Autodesk Inventor part; units mm, degrees
ref_plane "YZ Plane" through (0, 0, 0) normal (1, 0, 0) x (0, 1, 0)
ref_plane "XZ Plane" through (0, 0, 0) normal (0, 1, 0) x (-1, 0, 0)
ref_plane "XY Plane" through (0, 0, 0) normal (0, 0, 1) x (1, 0, 0)
sketch "Sketch1" plane through (0, 0, 0) normal (0, 0, 1) x (1, 0, 0)
  line L0 (-25.4, 25.4) -> (25.4, 25.4)
  line L1 (25.4, 25.4) -> (25.4, -25.4)
  line L2 (25.4, -25.4) -> (-25.4, -25.4)
  line L3 (-25.4, -25.4) -> (-25.4, 25.4)
  line L4 (23.2918, 23.2918) -> (-23.2918, 23.2918)
  line L5 (-23.2918, 23.2918) -> (-23.2918, -23.2918)
  line L6 (-23.2918, -23.2918) -> (23.2918, -23.2918)
  line L7 (23.2918, -23.2918) -> (23.2918, 23.2918)
  point P0 (0, 0)
  point P1 (23.2918, 0)
  point P2 (0, 25.4)
  dimension "d0" = 50.8
  dimension "d1" = 50.8
  dimension "d2" = 2.1082
extrude "Extrusion1" add sketch "Sketch1" along normal mid plane 914.4
properties part number "tube support base"
Source: CAD feature listing. Evaluate the final solid. Frame: model axes, mm. A direction names the side the tool comes from. Round coordinates to 2 decimals unless told otherwise and drop trailing zeros. Loops run counter-clockwise (first coordinate to the right, second up) from the corner with the lowest first, then second, coordinate; pieces in that order, holes last. Notation, with made-up numbers: M 77,-1 L 126,-1 A18 ccw 126,20 Z; hole C 4.5,7.25 d2. An arc over 180 degrees is marked long. Use a Markdown table: item, result. Add a question column.
1. Reachability of faces 4 (the flat face through (0, 25.4, -6)), 5 (the flat face through (0, 23.292, -6)) from +Z, -Z, +X, -X, +Y, -Y: full face, straight path, thin tool, end or side. Return the list, or none.
2. Line query: line 1 (Y direction, x = -14, z = 302). Output: solid intervals per line, ascending.
3. Mould query, pull axis Y, two halves, no side actions, for faces 1 (the flat face through (-2, -24, 457.2)), 2 (the flat face through (0, -23.292, -6)), 3 (the flat face through (0, -25.4, -6)). Classes: pulls with the +Y half, pulls with the -Y half, needs draft (parallel to the pull), parting line crosses it, or undercut.
4. Section query C-C on z = 379.5. Return the cut outline in (x, y).
5. Section query A-A on y = 12. Return the cut outline in (x, z), then the cut area to 3 significant figures.
Reported:
| question | item | result |
|---|---|---|
| 1 | face 4 | +Z, -Z, +X, -X, +Y |
| 1 | face 5 | +Z, -Z |
| 2 | line 1 | y = -25.4 to -23.29, 23.29 to 25.4 |
| 3 | face 1 | needs draft |
| 3 | face 2 | undercut |
| 3 | face 3 | pulls with the -Y half |
| 4 | outline | M -25.4,-25.4 L 25.4,-25.4 L 25.4,25.4 L -25.4,25.4 Z; hole M -23.29,-23.29 L 23.29,-23.29 L 23.29,23.29 L -23.29,23.29 Z |
| 5 | outline | M -25.4,-457.2 L -23.29,-457.2 L -23.29,457.2 L -25.4,457.2 Z; M 23.29,-457.2 L 25.4,-457.2 L 25.4,457.2 L 23.29,457.2 Z |
| 5 | area | 3,860 mm² |
